Could you check a few things on this model? Use its own coordinates, in mm. A direction names the side the tool comes from. Round coordinates to 2 decimals unless told otherwise and drop trailing zeros. Loops run counter-clockwise (first coordinate to the right, second up) from the corner with the lowest first, then second, coordinate; pieces in that order, holes last. Notation, with made-up numbers: M 7,39.25 L 58,39.25 A30 ccw 58,67.25 Z; hole C 52,-23 d11. An arc over 180 degrees is marked long. Answer in a Markdown table with one row per item.
```python
from build123d import *

# Parameters (mm, degrees)
F0_W          = 96
F0_H          = 78
F1_DEPTH      = 18
F2_W          = 72
F2_H          = 38
F3_DEPTH      = 58
F4_R          = 3
F5_W          = 72
F5_H          = 8
F6_DEPTH      = 12
F7_C1_SIZE    = 24
F8_SIZE2      = 14
F8_SIZE       = 36
F9_W          = 3
F9_H          = 14
F10_DEPTH     = 72
F11_W         = 20
F11_H         = 5
F12_DEPTH     = 96
F14_DEPTH     = 3
F16_DEPTH     = 16
F17_T1_DEPTH  = 72
F17_T3_DEPTH  = 32
F17_T5_DEPTH  = 46
F17_T8_ANGLE  = 180
F17_T10_ANGLE = 180
F17_T14_ANGLE = 233.2969892374
F17_T19_ANGLE = 233.2969892374
F17_T25_DEPTH = 39.5
F17_T29_DEPTH = 79.5
F17_T36_DEPTH = 79.5
F17_T40_DEPTH = 39.5
F17_T43_DEPTH = 22.5
F17_T45_DEPTH = 90
F17_T47_DEPTH = 72
F17_S51_W     = 3.06
F17_S51_H     = 3.06
F17_T52_DEPTH = 3.06
F17_S57_W     = 3.06
F17_S57_H     = 3.06
F17_T58_DEPTH = 3.06
F17_T62_ANGLE = 90
F17_T64_ANGLE = 90


# Not quite as in the source:
# - a fillet or chamfer that OpenCascade refuses, or shapes differently, is made with other operations: its cross-section is extruded or revolved along the edge and cut away or added


with BuildPart() as f1:
    # F0 (on Top) → F1 (new body)
    with BuildSketch(Plane.XY):
        with Locations((48, 39)):
            Rectangle(F0_W, F0_H)
    extrude(amount=F1_DEPTH)

    # F2 (on face) → F3 (join)
    with BuildSketch(Plane.XY.offset(18)):
        with Locations((48, 59)):
            Rectangle(F2_W, F2_H)
    extrude(amount=F3_DEPTH)

    # F4
    f4_edges = [f1.edges().sort_by_distance(p)[0] for p in [
        (90, 78, 18),
        (6, 78, 18),
    ]]
    fillet(f4_edges, radius=F4_R)

    # F5 (on face) → F6 (cut)
    with BuildSketch(Plane.XY.offset(76)):
        with Locations((48, 52)):
            Rectangle(F5_W, F5_H)
    extrude(amount=-F6_DEPTH, mode=Mode.SUBTRACT)

    # F7: chamfer of 24 on 2 edges, made by hand

    # F7_c1
    f7_c1_edges = [f1.edges().sort_by_distance(p)[0] for p in [
        (84, 44, 76),
    ]]
    chamfer(f7_c1_edges, length=F7_C1_SIZE)

    # F8
    f8_edges = [f1.edges().sort_by_distance(p)[0] for p in [
        (36, 78, 76),
    ]]
    f8_side = f1.faces().sort_by_distance((46.545455, 78, 34.461039))[0]
    chamfer(f8_edges, length=F8_SIZE, length2=F8_SIZE2, reference=f8_side)

    # F9 (on face) → F10 (cut, through all)
    with BuildSketch(Plane.YZ.offset(84)):
        with Locations((41.5, 25)):
            Rectangle(F9_W, F9_H)
    extrude(amount=-F10_DEPTH, mode=Mode.SUBTRACT)

    # F11 (on face) → F12 (cut, through all)
    with BuildSketch(Plane.YZ.offset(96)):
        with Locations((20, 2.5)):
            Rectangle(F11_W, F11_H)
    extrude(amount=-F12_DEPTH, mode=Mode.SUBTRACT)

    # F13 (on face) → F14 (join)
    with BuildSketch(Plane.XY.offset(18)):
        with BuildLine():
            ThreePointArc((71, 7), (84, 20), (71, 33))
            Line((71, 33), (25, 33))
            ThreePointArc((25, 33), (12, 20), (25, 7))
            Line((25, 7), (71, 7))
        make_face()
    extrude(amount=F14_DEPTH)

    # F15 (on face) → F16 (cut, through all)
    with BuildSketch(Plane.XY.offset(21)):
        with BuildLine():
            ThreePointArc((25, 26), (19, 20), (25, 14))
            Line((25, 14), (71, 14))
            ThreePointArc((71, 14), (77, 20), (71, 26))
            Line((71, 26), (25, 26))
        make_face()
    extrude(amount=-F16_DEPTH, mode=Mode.SUBTRACT)

    # F17: fillet of radius 3 on 17 edges, made by hand

    # F17_s2 → F17_t1 (join)
    with BuildSketch(Plane.YZ.offset(12)):
        with BuildLine():
            ThreePointArc((40, 32), (42.1213203436, 31.1213203436), (43, 29))
            Line((43, 29), (43, 32))
            Line((43, 32), (40, 32))
        make_face()
        with BuildLine():
            ThreePointArc((43, 21), (42.1213203436, 18.8786796564), (40, 18))
            Line((40, 18), (43, 18))
            Line((43, 18), (43, 21))
        make_face()
    extrude(amount=F17_T1_DEPTH)

    # F17_s4 → F17_t3 (join)
    with BuildSketch(Plane.XZ.offset(-75)):
        with BuildLine():
            ThreePointArc((84, 21), (84.8786796564, 18.8786796564), (87, 18))
            Line((87, 18), (84, 18))
            Line((84, 18), (84, 21))
        make_face()
        with BuildLine():
            ThreePointArc((9, 18), (11.1213203436, 18.8786796564), (12, 21))
            Line((12, 21), (12, 18))
            Line((12, 18), (9, 18))
        make_face()
    extrude(amount=F17_T3_DEPTH)

    # F17_s6 → F17_t5 (join)
    with BuildSketch(Plane.YZ.offset(25)):
        with BuildLine():
            ThreePointArc((4, 18), (6.1213203436, 18.8786796564), (7, 21))
            Line((7, 21), (7, 18))
            Line((7, 18), (4, 18))
        make_face()
        with BuildLine():
            ThreePointArc((36, 18), (33.8786796564, 18.8786796564), (33, 21))
            Line((33, 21), (33, 18))
            Line((33, 18), (36, 18))
        make_face()
    extrude(amount=F17_T5_DEPTH)

    # F17_s7 → F17_t8 (revolve)
    with BuildSketch(Plane.YZ.offset(25)):
        with BuildLine():
            ThreePointArc((36, 18), (33.8786796564, 18.8786796564), (33, 21))
            Line((33, 21), (33, 18))
            Line((33, 18), (36, 18))
        make_face()
    revolve(axis=Axis((25, 20, 18), (0, 0, 1)), revolution_arc=F17_T8_ANGLE)

    # F17_s9 → F17_t10 (revolve)
    with BuildSketch(Plane.YZ.offset(71)):
        with BuildLine():
            ThreePointArc((4, 18), (6.1213203436, 18.8786796564), (7, 21))
            Line((7, 21), (7, 18))
            Line((7, 18), (4, 18))
        make_face()
    revolve(axis=Axis((71, 20, 18), (0, 0, 1)), revolution_arc=F17_T10_ANGLE)


with BuildPart() as f17_tool12:
    # F17_s13 → F17_t14 (revolve)
    with BuildSketch(Plane(origin=(0, 19.6028186536, -26.2963148857), x_dir=(1, 0, 0), z_dir=(0, -0.5976672776, 0.8017442393))):
        with BuildLine():
            ThreePointArc((12, 63.0958271118), (11.1213203436, 65.2171474554), (9, 66.0958271118))
            Line((9, 66.0958271118), (12, 66.0958271118))
            Line((12, 66.0958271118), (12, 63.0958271118))
        make_face()
    revolve(axis=Axis((12, 75, 15), (1, 0, 0)), revolution_arc=F17_T14_ANGLE)

    split(bisect_by=Plane.XZ.offset(-78), keep=Keep.TOP)


with BuildPart() as f1_1:
    add(f1.part)

    # F17_t11: union F17_tool12
    add(f17_tool12.part)


with BuildPart() as f17_tool17:
    # F17_s18 → F17_t19 (revolve)
    with BuildSketch(Plane(origin=(0, 19.6028186536, -26.2963148857), x_dir=(1, 0, 0), z_dir=(0, -0.5976672776, 0.8017442393))):
        with BuildLine():
            ThreePointArc((84, 63.0958271118), (84.8786796564, 65.2171474554), (87, 66.0958271118))
            Line((87, 66.0958271118), (84, 66.0958271118))
            Line((84, 66.0958271118), (84, 63.0958271118))
        make_face()
    revolve(axis=Axis((84, 75, 15), (1, 0, 0)), revolution_arc=F17_T19_ANGLE)

    split(bisect_by=Plane.XZ.offset(-78), keep=Keep.TOP)


with BuildPart() as f1_2:
    add(f1_1.part)

    # F17_t16: union F17_tool17
    add(f17_tool17.part)


with BuildPart() as f17_tool23:
    # F17_s24 → F17_t25 (new body)
    with BuildSketch(Plane.XZ.offset(-35.5)):
        with BuildLine():
            ThreePointArc((84, 21), (84.8786796564, 18.8786796564), (87, 18))
            Line((87, 18), (84, 18))
            Line((84, 18), (84, 21))
        make_face()
    extrude(amount=-F17_T25_DEPTH)

    split(bisect_by=Plane.XZ.offset(-43), keep=Keep.TOP)


with BuildPart() as f17_tool27:
    # F17_s28 → F17_t29 (new body)
    with BuildSketch(Plane.YZ.offset(91.5)):
        with BuildLine():
            ThreePointArc((43, 21), (42.1213203436, 18.8786796564), (40, 18))
            Line((40, 18), (43, 18))
            Line((43, 18), (43, 21))
        make_face()
    extrude(amount=-F17_T29_DEPTH)

    split(bisect_by=Plane.YZ.offset(84), keep=Keep.TOP)


with BuildPart() as f17_tool23_1:
    add(f17_tool23.part)

    # F17_t31: intersect F17_tool27
    add(f17_tool27.part, mode=Mode.INTERSECT)


with BuildPart() as f1_3:
    add(f1_2.part)

    # F17_t21: union F17_tool23
    add(f17_tool23_1.part)


with BuildPart() as f17_tool34:
    # F17_s35 → F17_t36 (new body)
    with BuildSketch(Plane.YZ.offset(84)):
        with BuildLine():
            ThreePointArc((43, 21), (42.1213203436, 18.8786796564), (40, 18))
            Line((40, 18), (43, 18))
            Line((43, 18), (43, 21))
        make_face()
    extrude(amount=-F17_T36_DEPTH)

    split(bisect_by=Plane.YZ.offset(12), keep=Keep.BOTTOM)


with BuildPart() as f17_tool38:
    # F17_s39 → F17_t40 (new body)
    with BuildSketch(Plane.XZ.offset(-75)):
        with BuildLine():
            ThreePointArc((9, 18), (11.1213203436, 18.8786796564), (12, 21))
            Line((12, 21), (12, 18))
            Line((12, 18), (9, 18))
        make_face()
    extrude(amount=F17_T40_DEPTH)

    split(bisect_by=Plane.XZ.offset(-43), keep=Keep.TOP)


with BuildPart() as f17_tool34_1:
    add(f17_tool34.part)

    # F17_t42: intersect F17_tool38
    add(f17_tool38.part, mode=Mode.INTERSECT)


with BuildPart() as f1_4:
    add(f1_3.part)

    # F17_t32: union F17_tool34
    add(f17_tool34_1.part)

    # F17_s44 → F17_t43 (cut)
    with BuildSketch(Plane.XY.offset(-7.5)):
        with BuildLine():
            ThreePointArc((3, 0), (0.8786796564, 0.8786796564), (0, 3))
            Line((0, 3), (0, 0))
            Line((0, 0), (3, 0))
        make_face()
        with BuildLine():
            ThreePointArc((96, 3), (95.1213203436, 0.8786796564), (93, 0))
            Line((93, 0), (96, 0))
            Line((96, 0), (96, 3))
        make_face()
        with BuildLine():
            ThreePointArc((0, 75), (0.8786796564, 77.1213203436), (3, 78))
            Line((3, 78), (0, 78))
            Line((0, 78), (0, 75))
        make_face()
        with BuildLine():
            ThreePointArc((96, 75), (95.1213203436, 77.1213203436), (93, 78))
            Line((93, 78), (96, 78))
            Line((96, 78), (96, 75))
        make_face()
    extrude(amount=F17_T43_DEPTH, mode=Mode.SUBTRACT)

    # F17_s46 → F17_t45 (cut)
    with BuildSketch(Plane.YZ.offset(3)):
        with BuildLine():
            ThreePointArc((3, 18), (0.8786796564, 17.1213203436), (0, 15))
            Line((0, 15), (0, 18))
            Line((0, 18), (3, 18))
        make_face()
    extrude(amount=F17_T45_DEPTH, mode=Mode.SUBTRACT)

    # F17_s48 → F17_t47 (cut)
    with BuildSketch(Plane.XZ.offset(-75)):
        with BuildLine():
            ThreePointArc((3, 18), (0.8786796564, 17.1213203436), (0, 15))
            Line((0, 15), (0, 18))
            Line((0, 18), (3, 18))
        make_face()
        with BuildLine():
            ThreePointArc((93, 18), (95.1213203436, 17.1213203436), (96, 15))
            Line((96, 15), (96, 18))
            Line((96, 18), (93, 18))
        make_face()
    extrude(amount=F17_T47_DEPTH, mode=Mode.SUBTRACT)


with BuildPart() as f17_tool50:
    # F17_s51 → F17_t52 (new body)
    with BuildSketch(Plane.XY.offset(15)):
        with Locations((1.47, 1.47)):
            Rectangle(F17_S51_W, F17_S51_H)
    extrude(amount=F17_T52_DEPTH)

    # F17_s53 → F17_t54 (revolve, cut)
    with BuildSketch(Plane(origin=(3, 3, 15), x_dir=(0.7071067812, 0.7071067812, 0), z_dir=(0.7071067812, -0.7071067812, 0))):
        with BuildLine():
            ThreePointArc((0, -3), (3, 0), (0, 3))
            Line((0, 3), (0, -3))
        make_face()
    revolve(axis=Axis((3, 3, 15), (0, 0, 1)), mode=Mode.SUBTRACT)


with BuildPart() as f1_5:
    add(f1_4.part)

    # F17_t49: cut F17_tool50
    add(f17_tool50.part, mode=Mode.SUBTRACT)


with BuildPart() as f17_tool56:
    # F17_s57 → F17_t58 (new body)
    with BuildSketch(Plane.YZ.offset(93)):
        with Locations((1.47, 16.53)):
            Rectangle(F17_S57_W, F17_S57_H)
    extrude(amount=F17_T58_DEPTH)

    # F17_s59 → F17_t60 (revolve, cut)
    with BuildSketch(Plane(origin=(93, 3, 15), x_dir=(0, 0.7071067812, -0.7071067812), z_dir=(0, -0.7071067812, -0.7071067812))):
        with BuildLine():
            ThreePointArc((0, -3), (3, 0), (0, 3))
            Line((0, 3), (0, -3))
        make_face()
    revolve(axis=Axis((93, 3, 15), (1, 0, 0)), mode=Mode.SUBTRACT)


with BuildPart() as f1_6:
    add(f1_5.part)

    # F17_t55: cut F17_tool56
    add(f17_tool56.part, mode=Mode.SUBTRACT)

    # F17_s61 → F17_t62 (revolve, cut)
    with BuildSketch(Plane.XY.offset(15)):
        with BuildLine():
            ThreePointArc((93, 78), (95.1213203436, 77.1213203436), (96, 75))
            Line((96, 75), (96, 78))
            Line((96, 78), (93, 78))
        make_face()
    revolve(axis=Axis((96, 75, 15), (1, 0, 0)), revolution_arc=F17_T62_ANGLE, mode=Mode.SUBTRACT)

    # F17_s63 → F17_t64 (revolve, cut)
    with BuildSketch(Plane.XY.offset(15)):
        with BuildLine():
            ThreePointArc((0, 75), (0.8786796564, 77.1213203436), (3, 78))
            Line((3, 78), (0, 78))
            Line((0, 78), (0, 75))
        make_face()
    revolve(axis=Axis((0, 75, 15), (1, 0, 0)), revolution_arc=F17_T64_ANGLE, mode=Mode.SUBTRACT)


solid = f1_6.part
```
1) Which directions (+Z, -Z, +X, -X, +Y, -Y) give clear straight access to the entire face, cutting with the end or side of a thin tool? Please do faces 4 (the face through (48.55, 42.14, 18.9)), 5 (the face through (47.5, 42.1, 31.14)), 6 (the face through (84, 59, 36)).
Computed:
| item | result |
|---|---|
| face 4 | +X, -X |
| face 5 | +X, -X, -Y |
| face 6 | +Z, +X, +Y, -Y |
2) I want a section at D-D, the plane y = 50. Please give me the cut outline in (x, z).
Computed:
| item | result |
|---|---|
| outline | M 0,0 L 96,0 L 96,15 A3 ccw 93,18 L 87,18 A3 cw 84,21 L 84,52 L 72,64 L 12,64 L 12,21 A3 cw 9,18 L 3,18 A3 ccw 0,15 Z |
3) I want a section at A-A, the plane y = 20. Please give me the cut outline in (x, z).
Computed:
| item | result |
|---|---|
| outline | M 0,5 L 19,5 L 19,21 L 12,21 A3 cw 9,18 L 3,18 A3 ccw 0,15 Z; M 77,5 L 96,5 L 96,15 A3 ccw 93,18 L 87,18 A3 cw 84,21 L 77,21 Z |
4) Will these pins go through, and if not, where does the flat tip stop? P1, Ø1, axis at y = 67.5, z = 17.5, coming from the -X side; P2, Ø19, axis at y = 56.5, z = 45, coming from the -X side; P3, Ø2.5, axis at x = 33, z = 25, coming from the -Y side; P4, Ø21.5, axis at x = 53.5, y = 31, coming from the +Z side.
Computed:
| item | result |
|---|---|
| P1 | stops at x = 0.76 |
| P2 | stops at x = 12 |
| P3 | stops at y = 43 |
| P4 | stops at z = 76 |
5) I want a section at C-C, the plane z = 69.5. Please give me the cut outline in (x, y), plus the area to 3 significant figures.
Computed:
| item | result |
|---|---|
| outline | M 12,40 L 66.5,40 L 66.5,48 L 12,48 Z; M 12,56 L 66.5,56 L 66.5,66.53 L 12,66.53 Z |
| area | 1,010 mm² |
6) I need wall thicknesses on line 1 (Y direction, x = 49.5, z = 8.5); line 2 (X direction, y = 73, z = 25); line 3 (Z direction, x = 55.5, y = 52). Which ranges of each line are inside material? Lowest first, please.
Computed:
| item | result |
|---|---|
| line 1 | y = 0 to 14, 26 to 78 |
| line 2 | x = 12 to 84 |
| line 3 | z = 0 to 64 |
7) If we mould it in two halves opening along X, with no side actions, what happens to faces 1 (the face through (47.68, 6.1, 18.86)), 2 (the face through (0.9, 0.86, 7.4)), 3 (the face through (48, 14, 13))? For each: released by +X, released by -X, zero draft, split by the parting line, or undercut.
Computed:
| item | result |
|---|---|
| face 1 | zero draft |
| face 2 | released by -X |
| face 3 | undercut |
8) I want a section at B-B, the plane x = 68.5. Please give me the cut outline in (y, z), plus the area to 3 significant figures.
Computed:
| item | result |
|---|---|
| outline | M 0,0 L 10,0 L 10,5 L 14,5 L 14,21 L 7,21 A3 cw 4,18 L 3,18 A3 ccw 0,15 Z; M 26,5 L 30,5 L 30,0 L 78,0 L 78,40 L 67.31,67.5 L 56,67.5 L 56,64 L 48,64 L 48,67.5 L 40,67.5 L 40,32 A3 cw 43,29 L 43,21 A3 cw 40,18 L 36,18 A3 cw 33,21 L 26,21 Z |
| area | 2,860 mm² |
